Drawing for the job (mm, zero at the part's lowest x, y, z). A direction names the side the tool comes from. Round coordinates to 2 decimals unless told otherwise and drop trailing zeros. Loops run counter-clockwise (first coordinate to the right, second up) from the corner with the lowest first, then second, coordinate; pieces in that order, holes last. Notation, with made-up numbers: M 25,86.25 L 77,86.25 A21 ccw 77,103.25 Z; hole C -6.75,75 d8. An arc over 180 degrees is marked long. Use a Markdown table: item, result. Add a question column.
Q1. Cut at D-D (x = 30). Give the cut face in (y, z).
Q2. Tool access for the marked faces 1, 2, 3 and 4: list every direction of +Z, -Z, +X, -X, +Y, -Y with a clear straight run to the whole face (end or side of a thin tool).
Q3. Cut at B-B (x = 13). Give the cut face in (y, z).
Q4. Mould opens along Z. For the marked faces 5, 6 and 7 say: +Z half, -Z half, draft (parallel to the pull), parting line (faces both ways), or undercut.
Q5. Probe line 1 (Y direction, x = 18.5, z = 17.5); line 2 (Z direction, x = 37, y = 2.5); line 3 (Z direction, x = 12, y = 3.75). List the from-to ranges inside material, lowest first. Write a range as from..to.
Q6. Cut at C-C (z = 7.75). Give the cut face in (x, y), plus the area to 3 significant figures.
Q7. Pin check, flat tips, straight feed: pin 1 (0.6 mm diameter, centred on y = 4.5, z = 21, fed in from -X); pin 2 (1.2 mm diameter, centred on x = 21, y = 5.5, fed in from +Z); pin 3 (3 mm diameter, centred on y = 4, z = 11.5, fed in from +X). Stop position of each tip, or through.
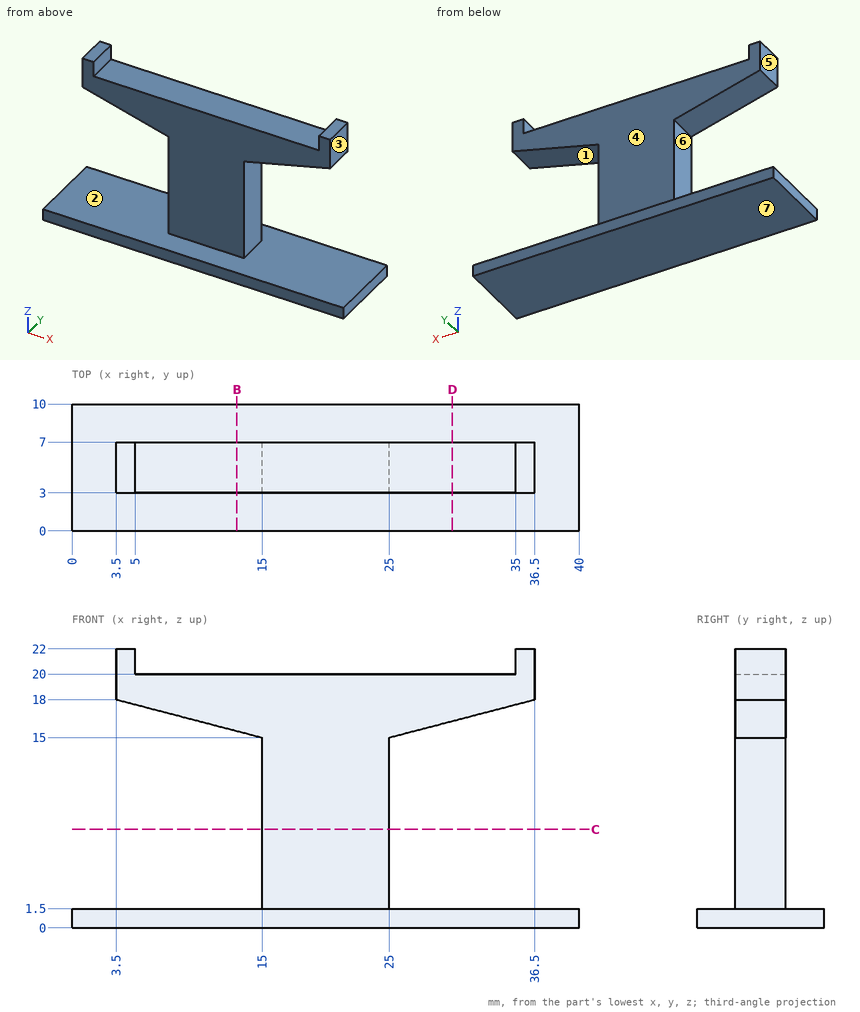
Checked values:
| question | item | result |
|---|---|---|
| 1 | outline | M 0,0 L 10,0 L 10,1.5 L 0,1.5 Z; M 3,16.3 L 7,16.3 L 7,20 L 3,20 Z |
| 2 | face 1 | +X, +Y, -Y |
| 2 | face 2 | none |
| 2 | face 3 | +Z, +X, +Y, -Y |
| 2 | face 4 | +Z, +X, -X, +Y |
| 3 | outline | M 0,0 L 10,0 L 10,1.5 L 0,1.5 Z; M 3,15.52 L 7,15.52 L 7,20 L 3,20 Z |
| 4 | face 5 | draft |
| 4 | face 6 | undercut |
| 4 | face 7 | -Z half |
| 5 | line 1 | y = 3..7 |
| 5 | line 2 | z = 0..1.5 |
| 5 | line 3 | z = 0..1.5, 15.78..20 |
| 6 | outline | M 15,3 L 25,3 L 25,7 L 15,7 Z |
| 6 | area | 40.0 mm^2 |
| 7 | pin 1 | stops at x = 3.5 |
| 7 | pin 2 | stops at z = 20 |
| 7 | pin 3 | stops at x = 25 |
